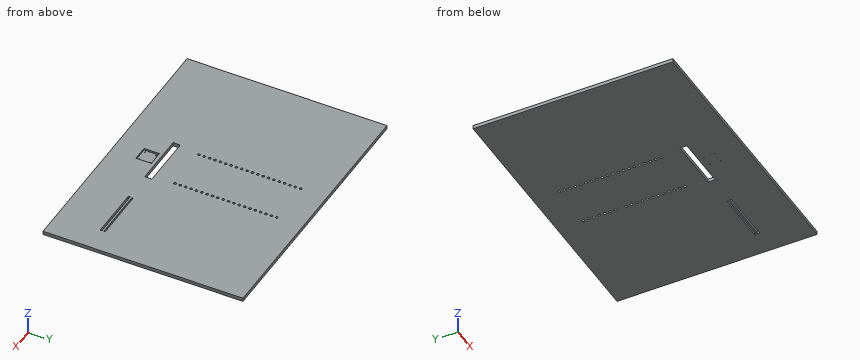
from build123d import *

# Parameters (mm, degrees)
F0_W      = 763
F0_H      = 560
F1_DEPTH  = 10
F2_R      = 3.5
F3_DEPTH  = 10
F4_W      = 43
F4_H      = 43
F4_R      = 1.5
F5_DEPTH  = 5
F6_DEPTH  = 10
F4_W_2    = 150
F4_H_2    = 20
F7_DEPTH  = 10
F8_DEPTH  = 10
F9_DEPTH  = 10
F10_DEPTH = 10


with BuildPart() as f1:
    # F0 (on Top) → F1 (new body)
    with BuildSketch(Plane.XY):
        Rectangle(F0_W, F0_H)
    extrude(amount=F1_DEPTH)

    # F2 (on face) → F3 (cut)
    with BuildSketch(Plane.XY.offset(10)):
        with Locations((-63.5, 206.5)):
            Circle(F2_R)
        with Locations((-63.5, 191.5)):
            Circle(F2_R)
        with Locations((-63.5, 176.5)):
            Circle(F2_R)
        with Locations((-63.5, 161.5)):
            Circle(F2_R)
        with Locations((-63.5, 146.5)):
            Circle(F2_R)
        with Locations((-63.5, 131.5)):
            Circle(F2_R)
        with Locations((-63.5, 116.5)):
            Circle(F2_R)
        with Locations((-63.5, 101.5)):
            Circle(F2_R)
        with Locations((-63.5, 86.5)):
            Circle(F2_R)
        with Locations((-63.5, 71.5)):
            Circle(F2_R)
        with Locations((-63.5, 56.5)):
            Circle(F2_R)
        with Locations((-63.5, 41.5)):
            Circle(F2_R)
        with Locations((-63.5, 26.5)):
            Circle(F2_R)
        with Locations((-63.5, 11.5)):
            Circle(F2_R)
        with Locations((-63.5, -3.5)):
            Circle(F2_R)
        with Locations((-63.5, -18.5)):
            Circle(F2_R)
        with Locations((-63.5, -33.5)):
            Circle(F2_R)
        with Locations((-63.5, -48.5)):
            Circle(F2_R)
        with Locations((-63.5, -63.5)):
            Circle(F2_R)
        with Locations((-63.5, -78.5)):
            Circle(F2_R)
        with Locations((63.5, 191.5)):
            Circle(F2_R)
        with Locations((63.5, 86.5)):
            Circle(F2_R)
        with Locations((63.5, 41.5)):
            Circle(F2_R)
        with Locations((63.5, 26.5)):
            Circle(F2_R)
        with Locations((63.5, 101.5)):
            Circle(F2_R)
        with Locations((63.5, -18.5)):
            Circle(F2_R)
        with Locations((63.5, 131.5)):
            Circle(F2_R)
        with Locations((63.5, -63.5)):
            Circle(F2_R)
        with Locations((63.5, 71.5)):
            Circle(F2_R)
        with Locations((63.5, 161.5)):
            Circle(F2_R)
        with Locations((63.5, 176.5)):
            Circle(F2_R)
        with Locations((63.5, -48.5)):
            Circle(F2_R)
        with Locations((63.5, 11.5)):
            Circle(F2_R)
        with Locations((63.5, -78.5)):
            Circle(F2_R)
        with Locations((63.5, -33.5)):
            Circle(F2_R)
        with Locations((63.5, 146.5)):
            Circle(F2_R)
        with Locations((63.5, -3.5)):
            Circle(F2_R)
        with Locations((63.5, 116.5)):
            Circle(F2_R)
        with Locations((63.5, 56.5)):
            Circle(F2_R)
        with Locations((63.5, 206.5)):
            Circle(F2_R)
    extrude(amount=-F3_DEPTH, mode=Mode.SUBTRACT)

    # F4 (on face) → F5 (cut)
    with BuildSketch(Plane.XY.offset(10)):
        with Locations((0, -188.5)):
            Rectangle(F4_W, F4_H)
        with Locations((-15.5, -204)):
            Circle(F4_R, mode=Mode.SUBTRACT)
        with Locations((-15.5, -173)):
            Circle(F4_R, mode=Mode.SUBTRACT)
        with Locations((15.5, -204)):
            Circle(F4_R, mode=Mode.SUBTRACT)
        with Locations((15.5, -173)):
            Circle(F4_R, mode=Mode.SUBTRACT)
    extrude(amount=-F5_DEPTH, mode=Mode.SUBTRACT)

    # F6 (cut): faces of the model
    f6_faces = [f1.faces().sort_by_distance(p)[0] for p in [
        (15.5, -204, 10),
        (15.5, -173, 10),
        (-15.5, -173, 10),
        (-15.5, -204, 10),
    ]]
    extrude(f6_faces, amount=-F6_DEPTH, mode=Mode.SUBTRACT)

    # F4 (on face) → F7 (cut)
    with BuildSketch(Plane.XY.offset(10)):
        with Locations((0, -147)):
            Rectangle(F4_W_2, F4_H_2)
    extrude(amount=-F7_DEPTH, mode=Mode.SUBTRACT)

    # F4 (on face) → F8 (cut)
    with BuildSketch(Plane.XY.offset(10)):
        with BuildLine():
            Line((309, -152), (164, -152))
            ThreePointArc((164, -152), (161.5, -154.5), (164, -157))
            Line((164, -157), (309, -157))
            ThreePointArc((309, -157), (311.5, -154.5), (309, -152))
        make_face()
    extrude(amount=-F8_DEPTH, mode=Mode.SUBTRACT)

    # F4 (on face) → F9 (cut)
    with BuildSketch(Plane.XY.offset(10)):
        with BuildLine():
            ThreePointArc((164.5, -143), (162.5, -145), (164.5, -147))
            Line((164.5, -147), (309.5, -147))
            ThreePointArc((309.5, -147), (311.5, -145), (309.5, -143))
            Line((309.5, -143), (164.5, -143))
        make_face()
    extrude(amount=-F9_DEPTH, mode=Mode.SUBTRACT)

    # F2 (on face) → F10 (cut)
    with BuildSketch(Plane.XY.offset(10)):
        with Locations((-63.5, 206.5)):
            Circle(F2_R)
        with Locations((-63.5, 191.5)):
            Circle(F2_R)
        with Locations((-63.5, 176.5)):
            Circle(F2_R)
        with Locations((-63.5, 161.5)):
            Circle(F2_R)
        with Locations((-63.5, 146.5)):
            Circle(F2_R)
        with Locations((-63.5, 131.5)):
            Circle(F2_R)
        with Locations((-63.5, 116.5)):
            Circle(F2_R)
        with Locations((-63.5, 101.5)):
            Circle(F2_R)
        with Locations((-63.5, 86.5)):
            Circle(F2_R)
        with Locations((-63.5, 71.5)):
            Circle(F2_R)
        with Locations((-63.5, 56.5)):
            Circle(F2_R)
        with Locations((-63.5, 41.5)):
            Circle(F2_R)
        with Locations((-63.5, 26.5)):
            Circle(F2_R)
        with Locations((-63.5, 11.5)):
            Circle(F2_R)
        with Locations((-63.5, -3.5)):
            Circle(F2_R)
        with Locations((-63.5, -18.5)):
            Circle(F2_R)
        with Locations((-63.5, -33.5)):
            Circle(F2_R)
        with Locations((-63.5, -48.5)):
            Circle(F2_R)
        with Locations((-63.5, -63.5)):
            Circle(F2_R)
        with Locations((-63.5, -78.5)):
            Circle(F2_R)
        with Locations((63.5, 191.5)):
            Circle(F2_R)
        with Locations((63.5, 86.5)):
            Circle(F2_R)
        with Locations((63.5, 41.5)):
            Circle(F2_R)
        with Locations((63.5, 26.5)):
            Circle(F2_R)
        with Locations((63.5, 101.5)):
            Circle(F2_R)
        with Locations((63.5, -18.5)):
            Circle(F2_R)
        with Locations((63.5, 131.5)):
            Circle(F2_R)
        with Locations((63.5, -63.5)):
            Circle(F2_R)
        with Locations((63.5, 71.5)):
            Circle(F2_R)
        with Locations((63.5, 161.5)):
            Circle(F2_R)
        with Locations((63.5, 176.5)):
            Circle(F2_R)
        with Locations((63.5, -48.5)):
            Circle(F2_R)
        with Locations((63.5, 11.5)):
            Circle(F2_R)
        with Locations((63.5, -78.5)):
            Circle(F2_R)
        with Locations((63.5, -33.5)):
            Circle(F2_R)
        with Locations((63.5, 146.5)):
            Circle(F2_R)
        with Locations((63.5, -3.5)):
            Circle(F2_R)
        with Locations((63.5, 116.5)):
            Circle(F2_R)
        with Locations((63.5, 56.5)):
            Circle(F2_R)
        with Locations((63.5, 206.5)):
            Circle(F2_R)
    extrude(amount=-F10_DEPTH, mode=Mode.SUBTRACT)


solid = f1.part
Geometry check sheet. Reference: the model listing, model coordinates, mm. Give positions to 0.01 mm unless a question says otherwise; leave off trailing zeros. Loops run counter-clockwise (first coordinate to the right, second up) from the corner with the lowest first, then second, coordinate; pieces in that order, holes last. Notation, with made-up numbers: M 61.25,37 L 90.25,37 A18 cw 90.25,48 Z; hole C 72,-38 d7. An arc over 180 degrees is marked long. Answer as a JSON object with one key per item and string values. Group by question number.
Item 1: Sectioned sample at C-C on z = 8.5. Give the number of separate pieces and of enclosed holes in the cut face, plus the area to 3 significant figures.
Item 2: Material ranges on L1, parallel to Y at x = 266, z = 5; L2, parallel to X at y = -204, z = 2.2; L3, parallel to Y at x = -36.5, z = 2.5, recorded low to high.
Item 3: Sectioned sample at A-A on x = 202.5. Record the boundary of the cut face in (y, z).
Item 4: Sectioned sample at B-B on x = 39. Record the boundary of the cut face in (y, z), plus the area to 3 significant figures.
Findings below:
{
 "1": {"separate pieces": "1", "enclosed holes": "44", "area": "420,000 mm2"},
 "2": {"L1": "-280 to -157, -152 to -147, -143 to 280", "L2": "-381.5 to -17, -14 to 14, 17 to 381.5", "L3": "-280 to -157, -137 to 280"},
 "3": {"outline": "M -280,0 L -157,0 L -157,10 L -280,10 Z; M -152,0 L -147,0 L -147,10 L -152,10 Z; M -143,0 L 280,0 L 280,10 L -143,10 Z"},
 "4": {"outline": "M -280,0 L -157,0 L -157,10 L -280,10 Z; M -137,0 L 280,0 L 280,10 L -137,10 Z", "area": "5,400 mm2"}
}
